For this review, use the dimensioned drawing (mm, ordinates from the lowest corner) and the shaded views. Coordinates: 2 decimals unless noted, no trailing zeros. Write each loop counter-clockwise with the first axis right and the second up, starting at its lowest first coordinate (ties: lowest second). Pieces come first, ordered by that corner, then holes. Notation, with made-up numbers: (15.5, 11) - (74.5, 11) arc R21 ccw to (74.5, 27) - close; hole circle Ø10 at (83, 72). An arc over 180 degrees is marked (long way). Use one line per item in the form item = value. Start each with the question number.
1) We need section D-D (z = 22.5). Give the boundary of the cut face in (x, y), plus the area to 3 significant figures.
2) We need section C-C (y = 1.6). Give the boundary of the cut face in (x, z).
3) We need section B-B (z = 10). Give the boundary of the cut face in (x, y), plus the area to 3 significant figures.
4) Insertion check: P1, Ø1.5, axis at x = 3, y = 2, coming from the +Z side; P2, Ø0.9, axis at y = 1, z = 33, coming from the -X side; P3, Ø0.9, axis at y = 1, z = 35.5, coming from the -X side. Each pin has a flat end and moves straight along its axis. Give the tip position at first contact, or say it passes through.
5) We need section A-A (x = 99.63). Give the boundary of the cut face in (y, z).
6) For L1, parallel to X at y = 1.45, z = 10; L2, parallel to Z at x = 72, y = 1.4; L3, parallel to Z at x = 106.5, y = 0.5, list the stretches that pass through material, from the lowest coordinate up. Write a range as from..to.
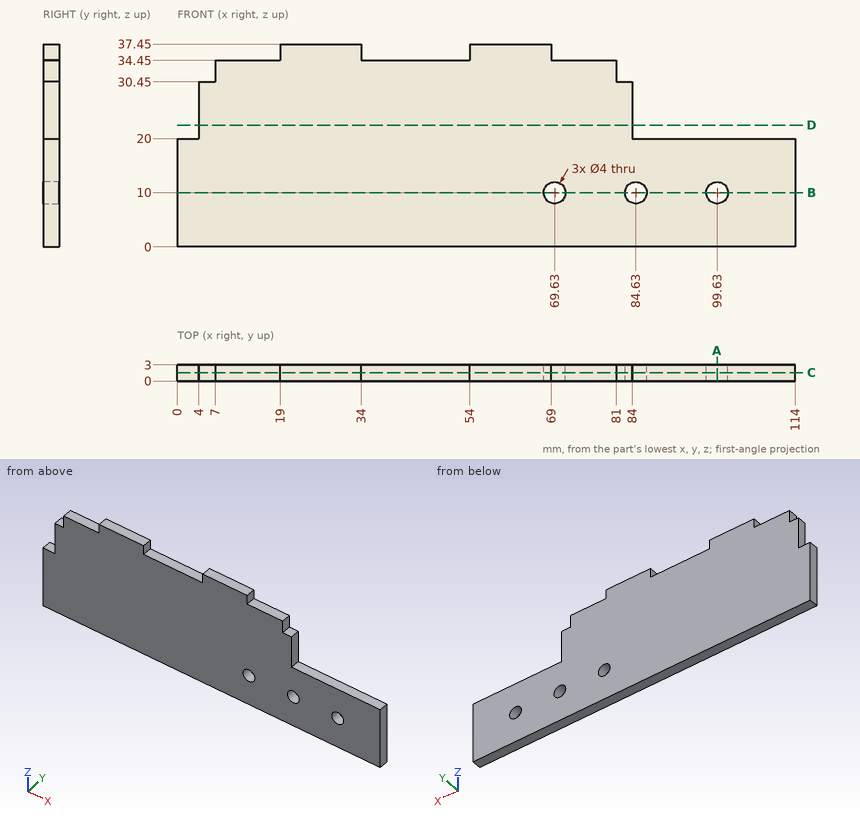
Determined:
q1.outline = (4, 0) - (84, 0) - (84, 3) - (4, 3) - close
q1.area = 240 mm²
q2.outline = (0, 0) - (114, 0) - (114, 20) - (84, 20) - (84, 30.45) - (81, 30.45) - (81, 34.45) - (69, 34.45) - (69, 37.45) - (54, 37.45) - (54, 34.45) - (34, 34.45) - (34, 37.45) - (19, 37.45) - (19, 34.45) - (7, 34.45) - (7, 30.45) - (4, 30.45) - (4, 20) - (0, 20) - close; hole circle Ø4 at (69.63, 10); hole circle Ø4 at (84.63, 10); hole circle Ø4 at (99.63, 10)
q3.outline = (0, 0) - (67.63, 0) - (67.63, 3) - (0, 3) - close; (71.63, 0) - (82.63, 0) - (82.63, 3) - (71.63, 3) - close; (86.63, 0) - (97.63, 0) - (97.63, 3) - (86.63, 3) - close; (101.63, 0) - (114, 0) - (114, 3) - (101.63, 3) - close
q3.area = 306 mm²
q4.P1 = 20
q4.P2 = 7
q4.P3 = 19
q5.outline = (0, 0) - (3, 0) - (3, 8) - (0, 8) - close; (0, 12) - (3, 12) - (3, 20) - (0, 20) - close
q6.L1 = 0..67.63, 71.63..82.63, 86.63..97.63, 101.63..114
q6.L2 = 0..34.45
q6.L3 = 0..20
